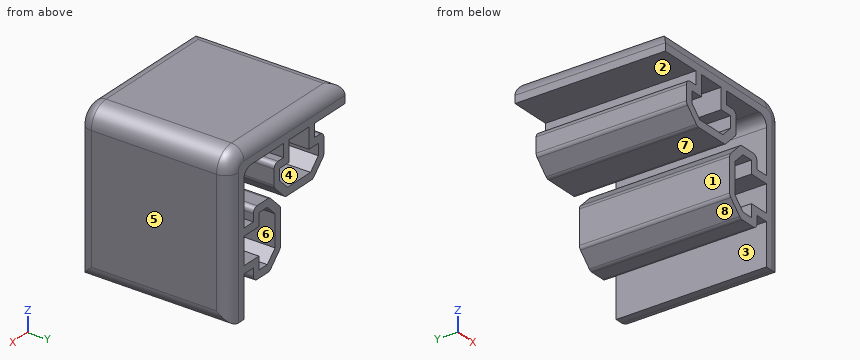
from build123d import *

# Parameters (mm, degrees)
BOSS_EXTRUDE1_DEPTH = 30
CUT_EXTRUDE3_REACH  = 51.163
SKETCH4_W           = 2.5
SKETCH4_H           = 30
CUT_EXTRUDE4_REACH  = 49.468
SKETCH5_W           = 2.5
SKETCH5_H           = 30
FILLET1_R           = 2.5
FILLET2_R           = 2
FILLET3_R           = 1
CUT_EXTRUDE5_REACH  = 42.274


with BuildPart() as part:
    # Sketch1 → Boss-Extrude1 (new body)
    with BuildSketch(Plane(origin=(0, 0, 0), x_dir=(1, 0, 0), z_dir=(0, 1, 0))):
        with BuildLine():
            Line((19, -15), (19, 15))
            Line((19, 15), (15, 15))
            Line((15, 15), (15, 4.2))
            Line((15, 4.2), (12.4, 4.2))
            Line((12.4, 4.2), (12.4, 6.75))
            Line((12.4, 6.75), (8, 6.75))
            Line((8, 6.75), (5, 3.75))
            Line((5, 3.75), (5, -3.75))
            Line((5, -3.75), (8, -6.75))
            Line((8, -6.75), (12.4, -6.75))
            Line((12.4, -6.75), (12.4, -4.2))
            Line((12.4, -4.2), (15, -4.2))
            Line((15, -4.2), (15, -15))
            Line((15, -15), (4.2, -15))
            Line((4.2, -15), (4.2, -12.4))
            Line((4.2, -12.4), (6.75, -12.4))
            Line((6.75, -12.4), (6.75, -8))
            Line((6.75, -8), (3.75, -5))
            Line((3.75, -5), (-3.75, -5))
            Line((-3.75, -5), (-6.75, -8))
            Line((-6.75, -8), (-6.75, -12.4))
            Line((-6.75, -12.4), (-4.2, -12.4))
            Line((-4.2, -12.4), (-4.2, -15))
            Line((-4.2, -15), (-15, -15))
            Line((-15, -15), (-15, -19))
            Line((-15, -19), (15, -19))
            ThreePointArc((15, -19), (17.828427125, -17.828427125), (19, -15))
        make_face()
    extrude(amount=BOSS_EXTRUDE1_DEPTH)

    # Sketch4 → Cut-Extrude3 (cut, up to next)
    with BuildSketch(Plane.XY.offset(19), mode=Mode.PRIVATE) as cut_extrude3_sk1:
        with Locations((-13.75, 15)):
            Rectangle(SKETCH4_W, SKETCH4_H)
    cut_extrude3_tool1 = extrude(cut_extrude3_sk1.sketch, amount=-CUT_EXTRUDE3_REACH, mode=Mode.PRIVATE) & part.part
    add(cut_extrude3_tool1.solids().sort_by_distance((-13.75, 15, 19))[0], mode=Mode.SUBTRACT)

    # Sketch5 → Cut-Extrude4 (cut, up to next)
    with BuildSketch(Plane(origin=(19, 0, 0), x_dir=(0, 0, -1), z_dir=(1, 0, 0)), mode=Mode.PRIVATE) as cut_extrude4_sk1:
        with Locations((13.75, 15)):
            Rectangle(SKETCH5_W, SKETCH5_H)
    cut_extrude4_tool1 = extrude(cut_extrude4_sk1.sketch, amount=-CUT_EXTRUDE4_REACH, mode=Mode.PRIVATE) & part.part
    add(cut_extrude4_tool1.solids().sort_by_distance((19, 15, -13.75))[0], mode=Mode.SUBTRACT)

    # Fillet1
    fillet1_edges = [part.edges().sort_by_distance(p)[0] for p in [
        (17.828427125, 30, 17.828427125),
        (19, 0, 1.25),
        (19, 30, 1.25),
        (19, 15, -12.5),
        (17.828427125, 0, 17.828427125),
        (1.25, 0, 19),
        (1.25, 30, 19),
        (-12.5, 15, 19),
    ]]
    fillet(fillet1_edges, radius=FILLET1_R)

    # Fillet2
    fillet2_edges = [part.edges().sort_by_distance(p)[0] for p in [
        (15, 15, 15),
    ]]
    fillet(fillet2_edges, radius=FILLET2_R)

    # Fillet3
    fillet3_edges = [part.edges().sort_by_distance(p)[0] for p in [
        (-6.75, 15, 12.4),
        (-6.75, 15, 8),
        (-3.75, 15, 5),
        (3.75, 15, 5),
        (6.75, 15, 8),
        (6.75, 15, 12.4),
        (12.4, 15, 6.75),
        (8, 15, 6.75),
        (5, 15, 3.75),
        (5, 15, -3.75),
        (8, 15, -6.75),
        (12.4, 15, -6.75),
    ]]
    fillet(fillet3_edges, radius=FILLET3_R)

    # Sketch6 → Cut-Extrude5 (cut, up to next)
    with BuildSketch(Plane(origin=(0, 30, 0), x_dir=(1, 0, 0), z_dir=(0, 1, 0)), mode=Mode.PRIVATE) as cut_extrude5_sk1:
        Polygon((5.25, -8.621320344), (3.128679656, -6.5), (-3.128679656, -6.5), (-5.25, -8.621320344), (-5.25, -10.9), (-2.7, -10.9), (-2.7, -15), (2.7, -15), (2.7, -10.9), (5.25, -10.9), align=None)
    cut_extrude5_tool1 = extrude(cut_extrude5_sk1.sketch, amount=-CUT_EXTRUDE5_REACH, mode=Mode.PRIVATE) & part.part
    # Sketch6 → Cut-Extrude5 (cut, up to next)
    with BuildSketch(Plane(origin=(0, 30, 0), x_dir=(1, 0, 0), z_dir=(0, 1, 0)), mode=Mode.PRIVATE) as cut_extrude5_sk2:
        Polygon((10.9, -2.7), (15, -2.7), (15, 2.7), (10.9, 2.7), (10.9, 5.25), (8.621320344, 5.25), (6.5, 3.128679656), (6.5, -3.128679656), (8.621320344, -5.25), (10.9, -5.25), align=None)
    cut_extrude5_tool2 = extrude(cut_extrude5_sk2.sketch, amount=-CUT_EXTRUDE5_REACH, mode=Mode.PRIVATE) & part.part
    add(cut_extrude5_tool1.solids().sort_by_distance((0, 30, 10.279151))[0], mode=Mode.SUBTRACT)
    add(cut_extrude5_tool2.solids().sort_by_distance((10.279151, 30, 0))[0], mode=Mode.SUBTRACT)


solid = part.part
CAD build for the part. Positions are in the model's coordinates, mm. Face numbers are marked on the shaded views. A direction names the side the tool comes from. Round coordinates to 2 decimals unless told otherwise and drop trailing zeros. Write each loop counter-clockwise with the first axis right and the second up, starting at its lowest first coordinate (ties: lowest second). Pieces come first, ordered by that corner, then holes. Notation, with made-up numbers: M -15,79 L -2,79 A17 ccw -2,97 Z; hole C 84,13 d3. An arc over 180 degrees is marked long. Use a Markdown table: item, result. Add a question column.
1. Slice it at B-B on z = -2. Give the cut face in (x, y), then the cut area to 3 significant figures.
2. Pull direction X, two halves, no side cores. Call the marked faces 5, 6, 7 and 8: released by +X, released by -X, zero draft, split by the parting line, or undercut.
3. 3-axis set-ups, long thin cutter, end or side, ignore diameter. For the marked faces 1, 2, 3 and 4: which of +Z, -Z, +X, -X, +Y, -Y reach the whole face in a straight line?
4. Drill centre lines: probe 1 along X at (y, z) = (27, 11); probe 2 along X at (y, z) = (23.5, 12.5); probe 3 along Z at (x, y) = (0, 11.75). Where is each one in solid material? Low to high.
5. Slice it at D-D on z = 14.5. Give the cut face in (x, y).
6. Slice it at A-A on x = -2. Give the cut face in (y, z), then the cut area to 3 significant figures.
7. Slice it at C-C on x = 13.5. Give the cut face in (y, z).
8. Flat gauge pins, fed straight in: P1, Ø2.5, axis at y = 12.5, z = 10, coming from the -X side; P2, Ø2, axis at y = 8, z = -0.5, coming from the -X side; P3, Ø3, axis at y = 13.5, z = 14, coming from the -X side; P4, Ø1.5, axis at x = 4, y = 10.5, coming from the -Z side. Where does each tip first touch, or does it go through?
Reply:
| question | item | result |
|---|---|---|
| 1 | outline | M 5,0 L 6.5,0 L 6.5,30 L 5,30 Z; M 15,0 L 16.5,0 A2.5 ccw 19,2.5 L 19,27.5 A2.5 ccw 16.5,30 L 15,30 Z |
| 1 | area | 162 mm^2 |
| 2 | face 5 | released by +X |
| 2 | face 6 | undercut |
| 2 | face 7 | zero draft |
| 2 | face 8 | released by -X |
| 3 | face 1 | -Z, -X, +Y, -Y |
| 3 | face 2 | -X, +Y, -Y |
| 3 | face 3 | -Z, +Y, -Y |
| 3 | face 4 | +Y, -Y |
| 4 | probe 1 | x = -6.75 to -2.7, 2.7 to 6.75, 15 to 19 |
| 4 | probe 2 | x = -4.2 to -2.7, 2.7 to 4.2, 15 to 19 |
| 4 | probe 3 | z = 5 to 6.5, 15 to 19 |
| 5 | outline | M -4.2,0 L -2.7,0 L -2.7,30 L -4.2,30 Z; M 2.7,0 L 4.2,0 L 4.2,30 L 2.7,30 Z; M 14.32,0 L 16.5,0 A2.5 ccw 19,2.5 L 19,27.5 A2.5 ccw 16.5,30 L 14.32,30 Z |
| 6 | outline | M 0,5 L 30,5 L 30,6.5 L 0,6.5 Z; M 0,15 L 30,15 L 30,16.5 A2.5 ccw 27.5,19 L 2.5,19 A2.5 ccw 0,16.5 Z |
| 6 | area | 162 mm^2 |
| 7 | outline | M 0,-4.2 L 30,-4.2 L 30,-2.7 L 0,-2.7 Z; M 0,2.7 L 30,2.7 L 30,4.2 L 0,4.2 Z; M 0,14.94 L 30,14.94 L 30,16.5 A2.5 ccw 27.5,19 L 2.5,19 A2.5 ccw 0,16.5 Z |
| 8 | P1 | stops at x = -6.75 |
| 8 | P2 | stops at x = 5 |
| 8 | P3 | stops at x = -12.5 |
| 8 | P4 | stops at z = 5 |
